Print and shaded views of the part. All mm, measured from the part's lowest x, y and z. Round coordinates to 2 decimals unless told otherwise and drop trailing zeros. Loops run counter-clockwise (first coordinate to the right, second up) from the corner with the lowest first, then second, coordinate; pieces in that order, holes last. Notation, with made-up numbers: (-25.5, -1) -> (-4.5, -1) arc R10 cw to (-4.5, 6) -> close; hole circle Ø7 at (51, 78). An arc over 180 degrees is marked (long way). Answer as CSV lines item,"result".
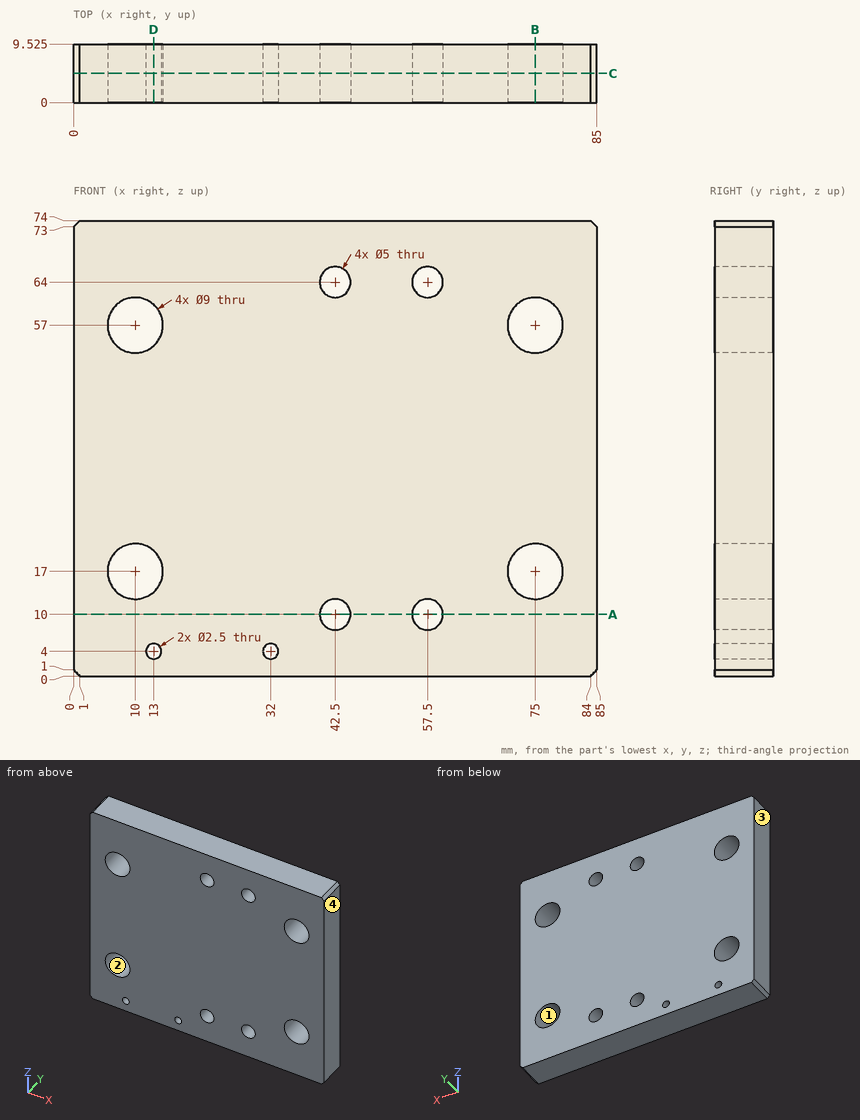
Q1. Slice it at D-D, the plane x = 13. Give the cut face in (y, z) (3 decimals).
Results:
outline,"(0, 0) -> (9.525, 0) -> (9.525, 2.75) -> (0, 2.75) -> close; (0, 5.25) -> (9.525, 5.25) -> (9.525, 13.646) -> (0, 13.646) -> close; (0, 20.354) -> (9.525, 20.354) -> (9.525, 53.646) -> (0, 53.646) -> close; (0, 60.354) -> (9.525, 60.354) -> (9.525, 74) -> (0, 74) -> close"
Q2. Slice it at A-A, the plane z = 10. Give the cut face in (x, y) (3 decimals).
Results:
outline,"(0, 0) -> (40, 0) -> (40, 9.525) -> (0, 9.525) -> close; (45, 0) -> (55, 0) -> (55, 9.525) -> (45, 9.525) -> close; (60, 0) -> (85, 0) -> (85, 9.525) -> (60, 9.525) -> close"
Q3. Two-plate mould, pull along X, no slides. Class the marked faces 1, 2, 3 and 4: pulls with the +X half, pulls with the -X half, needs draft (parallel to the pull), parting line crosses it, or undercut.
Results:
face 1,"undercut"
face 2,"undercut"
face 3,"pulls with the -X half"
face 4,"pulls with the +X half"
Q4. Slice it at B-B, the plane x = 75. Give the cut face in (y, z) (3 decimals), and give its area (3 significant figures).
Results:
outline,"(0, 0) -> (9.525, 0) -> (9.525, 12.5) -> (0, 12.5) -> close; (0, 21.5) -> (9.525, 21.5) -> (9.525, 52.5) -> (0, 52.5) -> close; (0, 61.5) -> (9.525, 61.5) -> (9.525, 74) -> (0, 74) -> close"
area,"533 mm2"
Q5. Probe L1, parallel to Z at x = 75, y = 6; L2, parallel to X at y = 5.75, z = 64; L3, parallel to Z at x = 57.5, y = 4.25. List the from-to ranges inside material, lowest first. Write a range as [from, to].
Results:
L1,"[0, 12.5], [21.5, 52.5], [61.5, 74]"
L2,"[0, 40], [45, 55], [60, 85]"
L3,"[0, 7.5], [12.5, 61.5], [66.5, 74]"
Q6. Slice it at C-C, the plane y = 4.75. Count the separate pieces of the cut face and the enclosed holes in it, and give its area (3 significant figures).
Results:
separate pieces,"1"
enclosed holes,"10"
area,"5,950 mm2"
Q7. Drop a flat-ended pin along its axis: pin 1 Ø4.5 at (x, z) = (57.5, 64) entering from -Y. Give the stop position or say it passes through.
Results:
pin 1,"through"
